Read the model definition and answer for the solid it produces. Units are mm, in the model's axes. A direction names the side the tool comes from. Round coordinates to 2 decimals unless told otherwise and drop trailing zeros. Order: outer loops, then holes, each group sorted by start corner. A loop starts at its lowest first (then second) coordinate and runs counter-clockwise, first axis right, second up. Notation, with made-up numbers: (40, -12.75) - (58, -12.75) arc R15 ccw to (58, -2.75) - close; hole circle Ø10 at (55.25, -26). An arc over 180 degrees is marked (long way). Put each result on its own line as item: value. Start each with the question number.
Q1. For a pull along X with two mould halves and no side action, classify faces 4 (the face through (3, 1.5, 1)), 5 (the face through (-2, 1, -4)), 6 (the face through (-4.88, 0.02, -1.08)) as pulls with the +X half, pulls with the -X half, needs draft (parallel to the pull), parting line crosses it, or undercut.
Q2. Which of the six approach directions +Z, -Z, +X, -X, +Y, -Y give full straight-line access (tool end or side, diameter ignored) to faces 1 (the face through (0.9, -0.02, 2.86)), 2 (the face through (-3.905, 1.254, -0.867)), 3 (the face through (-2.89, -1.25, -3.77))?
Q3. Section A-A on z = 0 is taken. Give the vertices of the cut face in (x, y).
Q4. This flat-tipped pin is pushed along its axis until it touches: pin 1 Ø5 at (x, z) = (0, 1.5) entering from +Y. Where does it stop, or does it pass through?
Q5. Section B-B on x = 0 is taken. Give the vertices of the cut face in (y, z), then the cut area to 3 significant figures.
Q6. Section C-C on z = 3.75 is taken. Give the vertices of the cut face in (x, y).
Q7. Find the intervals of material crossed by line 1 along X through (y, z) = (-1.15, 0); line 2 along Y through (x, z) = (-1, -4.5); line 3 along X through (y, z) = (0.8, 0), in increasing order. Write a range as from..to.
Q8. Section D-D on y = 0.6 is taken. Give the vertices of the cut face in (x, z).
from build123d import *

# Parameters (mm, degrees)
SKETCH_1_R        = 5
SKETCH_1_R_2      = 4.75
EXTRUDE_1_DEPTH   = 1.5
SKETCH_1_R_3      = 4
SKETCH_1_R_4      = 3
EXTRUDE_1_2_DEPTH = 1.5
SKETCH_1_3_R      = 4.75
SKETCH_1_3_R_2    = 4
EXTRUDE_2_DEPTH   = 1


with BuildPart() as part:
    # Sketch 1 → Extrude 1 (new, symmetric)
    with BuildSketch(Plane(origin=(0, 0, 0), x_dir=(1, 0, 0), z_dir=(0, 1, 0))):
        with Locations(Location((0, 0, 0), (0, 0, 270))):
            Circle(SKETCH_1_R)
        with Locations(Location((0, 0, 0), (0, 0, 270))):
            Circle(SKETCH_1_R_2, mode=Mode.SUBTRACT)
    extrude(amount=EXTRUDE_1_DEPTH, both=True)



with BuildPart() as body_2:
    # Sketch 1 → Extrude 1 2 (new, symmetric)
    with BuildSketch(Plane(origin=(0, 0, 0), x_dir=(1, 0, 0), z_dir=(0, 1, 0))):
        with Locations(Location((0, 0, 0), (0, 0, 270))):
            Circle(SKETCH_1_R_3)
        with Locations(Location((0, 0, 0), (0, 0, 270))):
            Circle(SKETCH_1_R_4, mode=Mode.SUBTRACT)
    extrude(amount=EXTRUDE_1_2_DEPTH, both=True)


with BuildPart() as part_1:
    add(part.part)

    add(body_2.part)  # Extrude 2 merges body 2
    # Sketch 1_3 → Extrude 2 (add, symmetric)
    with BuildSketch(Plane(origin=(0, 0, 0), x_dir=(1, 0, 0), z_dir=(0, 1, 0))):
        with Locations(Location((0, 0, 0), (0, 0, 270))):
            Circle(SKETCH_1_3_R)
        with Locations(Location((0, 0, 0), (0, 0, 270))):
            Circle(SKETCH_1_3_R_2, mode=Mode.SUBTRACT)
    extrude(amount=EXTRUDE_2_DEPTH, both=True)


solid = part_1.part
Findings:
1. face 4: needs draft
1. face 5: undercut
1. face 6: parting line crosses it
2. face 1: +Y, -Y
2. face 2: +Y
2. face 3: -Y
3. outline: (-5, -1.5) - (-4.75, -1.5) - (-4.75, -1) - (-4, -1) - (-4, -1.5) - (-3, -1.5) - (-3, 1.5) - (-4, 1.5) - (-4, 1) - (-4.75, 1) - (-4.75, 1.5) - (-5, 1.5) - close; (3, -1.5) - (4, -1.5) - (4, -1) - (4.75, -1) - (4.75, -1.5) - (5, -1.5) - (5, 1.5) - (4.75, 1.5) - (4.75, 1) - (4, 1) - (4, 1.5) - (3, 1.5) - close
4. pin 1: y = 1.5
5. outline: (-1.5, -5) - (1.5, -5) - (1.5, -4.75) - (1, -4.75) - (1, -4) - (1.5, -4) - (1.5, -3) - (-1.5, -3) - (-1.5, -4) - (-1, -4) - (-1, -4.75) - (-1.5, -4.75) - close; (-1.5, 3) - (1.5, 3) - (1.5, 4) - (1, 4) - (1, 4.75) - (1.5, 4.75) - (1.5, 5) - (-1.5, 5) - (-1.5, 4.75) - (-1, 4.75) - (-1, 4) - (-1.5, 4) - close
5. area: 10.5 mm2
6. outline: (-3.31, -1.5) - (-2.92, -1.5) - (-2.92, -1) - (-1.39, -1) - (-1.39, -1.5) - (1.39, -1.5) - (1.39, -1) - (2.92, -1) - (2.92, -1.5) - (3.31, -1.5) - (3.31, 1.5) - (2.92, 1.5) - (2.92, 1) - (1.39, 1) - (1.39, 1.5) - (-1.39, 1.5) - (-1.39, 1) - (-2.92, 1) - (-2.92, 1.5) - (-3.31, 1.5) - close
7. line 1: -5..-4.75, -4..-3, 3..4, 4.75..5
7. line 2: -1..1
7. line 3: -5..-3, 3..5
8. outline: circle Ø10 at (0, 0); hole circle Ø6 at (0, 0)
